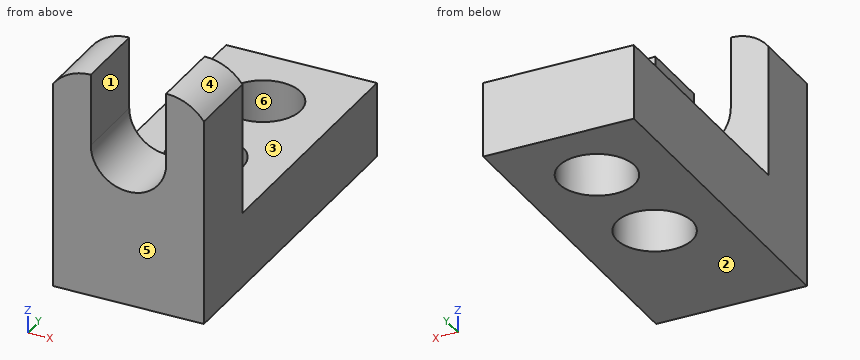
from build123d import *

# Parameters (mm, degrees)
F1_DEPTH = 25.4
F3_DEPTH = 25.4
F5_DEPTH = 25.4
F7_DEPTH = 25.4
F8_R     = 6.35
F9_DEPTH = 25.4


with BuildPart() as f1:
    # F0 (on Right) → F1 (new body)
    with BuildSketch(Plane.YZ):
        Polygon((0, 38.1), (0, 0), (57.15, 0), (57.15, 12.7), (12.7, 12.7), (12.7, 38.1), align=None)
    extrude(amount=F1_DEPTH)

    # F2 (on face) → F3 (cut)
    with BuildSketch(Plane(origin=(0, 12.7, 0), x_dir=(-1, 0, 0), z_dir=(0, 1, 0))):
        with BuildLine():
            ThreePointArc((-19.05, 25.8947107941), (-12.7, 19.5447107941), (-6.35, 25.8947107941))
            ThreePointArc((-6.35, 25.8947107941), (-12.7, 32.2447107941), (-19.05, 25.8947107941))
        make_face()
        with BuildLine():
            ThreePointArc((-19.05, 25.8947107941), (-12.7, 32.2447107941), (-6.35, 25.8947107941))
            Line((-6.35, 25.8947107941), (-6.35, 38.1))
            Line((-6.35, 38.1), (-19.05, 38.1))
            Line((-19.05, 38.1), (-19.05, 25.8947107941))
        make_face()
    extrude(amount=-F3_DEPTH, mode=Mode.SUBTRACT)

    # F4 (on face) → F5 (cut)
    with BuildSketch(Plane(origin=(0, 12.7, 0), x_dir=(-1, 0, 0), z_dir=(0, 1, 0))):
        with BuildLine():
            ThreePointArc((-25.4, 34.925), (-22.5997579143, 37.2620158286), (-19.05, 38.1))
            Line((-19.05, 38.1), (-25.4, 38.1))
            Line((-25.4, 38.1), (-25.4, 34.925))
        make_face()
    extrude(amount=-F5_DEPTH, mode=Mode.SUBTRACT)

    # F6 (on face) → F7 (cut)
    with BuildSketch(Plane(origin=(0, 12.7, 0), x_dir=(-1, 0, 0), z_dir=(0, 1, 0))):
        with BuildLine():
            ThreePointArc((-6.35, 38.1), (-2.8002420857, 37.2620158286), (0, 34.925))
            Line((0, 34.925), (0, 38.1))
            Line((0, 38.1), (-6.35, 38.1))
        make_face()
    extrude(amount=-F7_DEPTH, mode=Mode.SUBTRACT)

    # F8 (on face) → F9 (cut)
    with BuildSketch(Plane.XY.offset(12.7)):
        with Locations((12.7, 44.45)):
            Circle(F8_R)
        with Locations((12.7, 25.4)):
            Circle(F8_R)
    extrude(amount=-F9_DEPTH, mode=Mode.SUBTRACT)


solid = f1.part
Input: part model. Units: mm. Frame: model coordinates. Face numbers are marked on the shaded views. A direction names the side the tool comes from. Give positions to 0.01 mm unless a question says otherwise; leave off trailing zeros. Loops run counter-clockwise (first coordinate to the right, second up) from the corner with the lowest first, then second, coordinate; pieces in that order, holes last. Notation, with made-up numbers: M -31,23 L 7,23 A16 cw 7,53 Z; hole C 3,49 d4. An arc over 180 degrees is marked long. Use CSV: the item, a comma, the result in double quotes.
(1) Pull-direction query (Y, two-part tool) for the marked faces 4, 5 and 6; classes: pulls with the +Y half, pulls with the -Y half, needs draft (parallel to the pull), parting line crosses it, or undercut.
Outcome:
face 4,"needs draft"
face 5,"pulls with the -Y half"
face 6,"undercut"
(2) Section A-A, the plane x = 12.7. Return loops of the section in (y, z), plus the area to 3 significant figures.
Outcome:
outline,"M 0,0 L 19.05,0 L 19.05,12.7 L 12.7,12.7 L 12.7,19.54 L 0,19.54 Z; M 31.75,0 L 38.1,0 L 38.1,12.7 L 31.75,12.7 Z; M 50.8,0 L 57.15,0 L 57.15,12.7 L 50.8,12.7 Z"
area,"490 mm²"
(3) Section C-C, the plane z = 7. Return loops of the section in (x, y).
Outcome:
outline,"M 0,0 L 25.4,0 L 25.4,57.15 L 0,57.15 Z; hole C 12.7,25.4 d12.7; hole C 12.7,44.45 d12.7"
(4) Pin query (flat end, axial travel): P1, Ø1.5, axis at x = 3.5, z = 14, coming from the +Y side; P2, Ø6, axis at x = 18, y = 48.5, coming from the +Z side. Return the tip coordinate at first contact, or that it passes through.
Outcome:
P1,"stops at y = 12.7"
P2,"stops at z = 12.7"
(5) Section D-D, the plane z = 24.5. Return loops of the section in (x, y).
Outcome:
outline,"M 0,0 L 6.51,0 L 6.51,12.7 L 0,12.7 Z; M 18.89,0 L 25.4,0 L 25.4,12.7 L 18.89,12.7 Z"
(6) Set-up query: the marked faces 1, 2 and 3. Return all of +Z, -Z, +X, -X, +Y, -Y with unobstructed straight access to the full face (end or side cutting, diameter ignored); none if empty.
Outcome:
face 1,"+Z, +Y, -Y"
face 2,"-Z, +X, -X, +Y, -Y"
face 3,"+Z, +X, -X, +Y"
(7) Material intervals for L1, parallel to Y at x = 12.7, z = 8.5; L2, parallel to X at y = 25, z = 4; L3, parallel to Y at x = 7.5, z = 11, sorted ascending. Write a range as [from, to].
Outcome:
L1,"y = [0, 19.05], [31.75, 38.1], [50.8, 57.15]"
L2,"x = [0, 6.36], [19.04, 25.4]"
L3,"y = [0, 21.76], [29.04, 40.81], [48.09, 57.15]"
(8) Section B-B, the plane y = 25.4. Return loops of the section in (x, z).
Outcome:
outline,"M 0,0 L 6.35,0 L 6.35,12.7 L 0,12.7 Z; M 19.05,0 L 25.4,0 L 25.4,12.7 L 19.05,12.7 Z"
